Design review of the part built by this model. Coordinates are the model's own, in mm. Face numbers are marked on the shaded views. A direction names the side the tool comes from. Give positions to 0.01 mm unless a question says otherwise; leave off trailing zeros. Write each question's results on one line, items separated by ' | '. Start each with the question number.
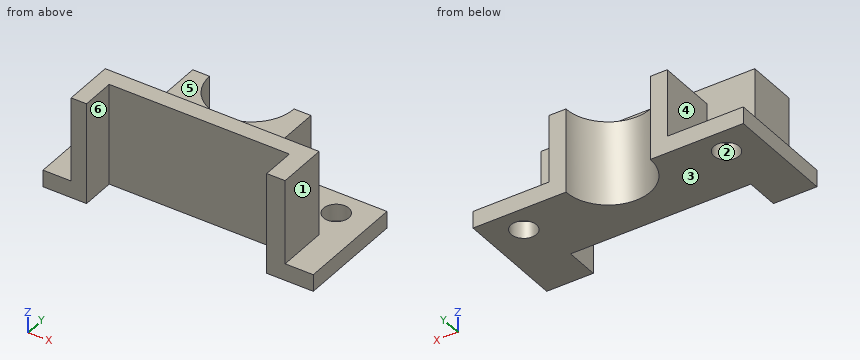
Autodesk Inventor part; units mm, degrees
ref_plane "YZ Plane" through (0, 0, 0) normal (1, 0, 0) x (0, 1, 0)
ref_plane "XZ Plane" through (0, 0, 0) normal (0, 1, 0) x (-1, 0, 0)
ref_plane "XY Plane" through (0, 0, 0) normal (0, 0, 1) x (1, 0, 0)
sketch "Boceto1" plane through (0, 0, 0) normal (0, 0, 1) x (1, 0, 0)
  line L0 (0, 0) -> (152.4, 0)
  line L1 (152.4, 0) -> (152.4, 61.9125)
  line L2 (152.4, 61.9125) -> (0, 61.9125)
  line L3 (0, 61.9125) -> (0, 0)
  dimension "d0" = 152.4
  dimension "d1" = 61.9125
extrude "Bloque_Posterior" add sketch "Boceto1" along normal blind 9.525
sketch "Boceto2" plane through (0, 0, 9.525) normal (0, 0, 1) x (1, 0, 0)
  line L0 (15.875, 0) -> (136.525, 0)
  line L1 (136.525, 0) -> (136.525, 28.575)
  line L2 (136.525, 28.575) -> (15.875, 28.575)
  line L3 (15.875, 28.575) -> (15.875, 0)
  line L4 (0, 0) -> (152.4, 0)
  line L5 (76.2, 0) -> (76.2, 70.6909) construction
  dimension "d4" = 120.65
  dimension "d5" = 28.575
  dimension "d6" = 60.325
extrude "Bloque_Inferior" add sketch "Boceto2" along normal blind 47.625
sketch "Boceto3" plane through (0, 0, 9.525) normal (0, 0, 1) x (1, 0, 0)
  line L0 (0, 0) -> (152.4, 0)
  line L1 (76.2, 0) -> (76.2, 86.7708) construction
  line L2 (42.8625, 61.9125) -> (109.5375, 61.9125)
  line L3 (109.5375, 61.9125) -> (109.5375, 28.575)
  line L4 (109.5375, 28.575) -> (42.8625, 28.575)
  line L5 (42.8625, 28.575) -> (42.8625, 61.9125)
  line L6 (152.4, 61.9125) -> (0, 61.9125)
  dimension "d9" = 66.675
  dimension "d10" = 33.3375
  dimension "d11" = 33.3375
extrude "Bloque_Superior" add sketch "Boceto3" along normal blind 38.1
sketch "Boceto4" plane through (0, 0, 9.525) normal (0, 0, 1) x (1, 0, 0)
  line L0 (0, 0) -> (152.4, 0)
  line L1 (24.5425, 0) -> (126.1425, 0)
  line L2 (126.1425, 0) -> (126.1425, 19.05)
  line L3 (126.1425, 19.05) -> (24.5425, 19.05)
  line L4 (24.5425, 19.05) -> (24.5425, 0)
  dimension "d14" = 101.6
  dimension "d15" = 19.05
extrude "Orificio_Inferior" cut sketch "Boceto4" along normal blind 47.625 and the other way blind 23.8252
sketch "Boceto5" plane through (0, 0, 47.625) normal (0, 0, 1) x (1, 0, 0)
  line L0 (109.5375, 61.9125) -> (42.8625, 61.9125)
  arc A0 (52.3875, 61.9125) -> (100.0125, 61.9125) centre (76.2, 61.9125) ccw
  point P0 (0, 0)
  dimension "d20" = 47.625
extrude "Agujero_Central" cut sketch "Boceto5" against normal blind 47.625
sketch "Boceto6" plane through (0, 0, 9.525) normal (0, 0, 1) x (1, 0, 0)
  line L0 (-22.923, 47.625) -> (163.4069, 47.625) construction
  line L1 (19.05, -6.8102) -> (19.05, 78.4252) construction
  line L2 (42.8625, 61.9125) -> (0, 61.9125)
  line L3 (0, 61.9125) -> (0, 0)
  circle A0 centre (19.05, 47.625) radius 7.1437
  dimension "d23" = 14.2875
  dimension "d24" = 19.05
  dimension "d25" = 14.2875
extrude "Agujero_Izquierdo" cut sketch "Boceto6" against normal blind 9.525
sketch "Boceto7" plane through (0, 0, 9.525) normal (0, 0, 1) x (1, 0, 0)
  line L0 (133.35, 81.3516) -> (133.35, -20.5289) construction
  line L1 (173.8284, 47.625) -> (-5.5853, 47.625) construction
  line L2 (152.4, 0) -> (152.4, 61.9125)
  line L3 (152.4, 61.9125) -> (109.5375, 61.9125)
  circle A0 centre (133.35, 47.625) radius 7.1438
  point P0 (0, 0)
  dimension "d28" = 19.05
  dimension "d29" = 14.2875
  dimension "d30" = 14.2875
extrude "Agujero_Derecho" cut sketch "Boceto7" against normal blind 9.525
Q1. Add section C-C on z = 4. Count the separate pieces of the cut face and the enclosed holes in it, plus the area to 3 significant figures.
Q2. Insertion check: P1, Ø9.5, axis at y = 7, z = 34, coming from the +X side (3 decimals); P2, Ø8, axis at y = 36.5, z = 45, coming from the +X side; P3, Ø21, axis at y = 9, z = 37, coming from the -X side (3 decimals). Each pin has a flat end and moves straight along its axis. Give the tip position at first contact, or say it passes through.
Q3. For line 1 along X through (y, z) = (13.5, 44.5) (1 decimal); line 2 along Y through (x, z) = (133.35, 7); line 3 along X through (y, z) = (36.5, 34.5), list the stretches that pass through material, from the lowest coordinate up. Write a range as [from, to].
Q4. The part is to be moulded in two halves that separate along X. For the marked faces 1, 2 and 3, say which applies: +X half, -X half, draft (parallel to the pull), parting line (faces both ways), or undercut.
Q5. Machinability: for the marked faces 4, 5 and 6, which of the approach directions +Z, -Z, +X, -X, +Y, -Y give a long, thin tool a straight path to every point of the face, cutting with its end or side? Answer none if there is none.
Result:
1) separate pieces: 1 | enclosed holes: 2 | area: 6,290 mm²
2) P1: stops at x = 136.525 | P2: stops at x = 109.54 | P3: stops at x = 15.875
3) line 1: x = [15.9, 24.5], [126.1, 136.5] | line 2: y = [0, 40.48], [54.77, 61.91] | line 3: x = [42.86, 109.54]
4) face 1: +X half | face 2: undercut | face 3: draft
5) face 4: +Z, -X, +Y | face 5: +Z, +X, -X, +Y | face 6: +Z, -Z, -Y
